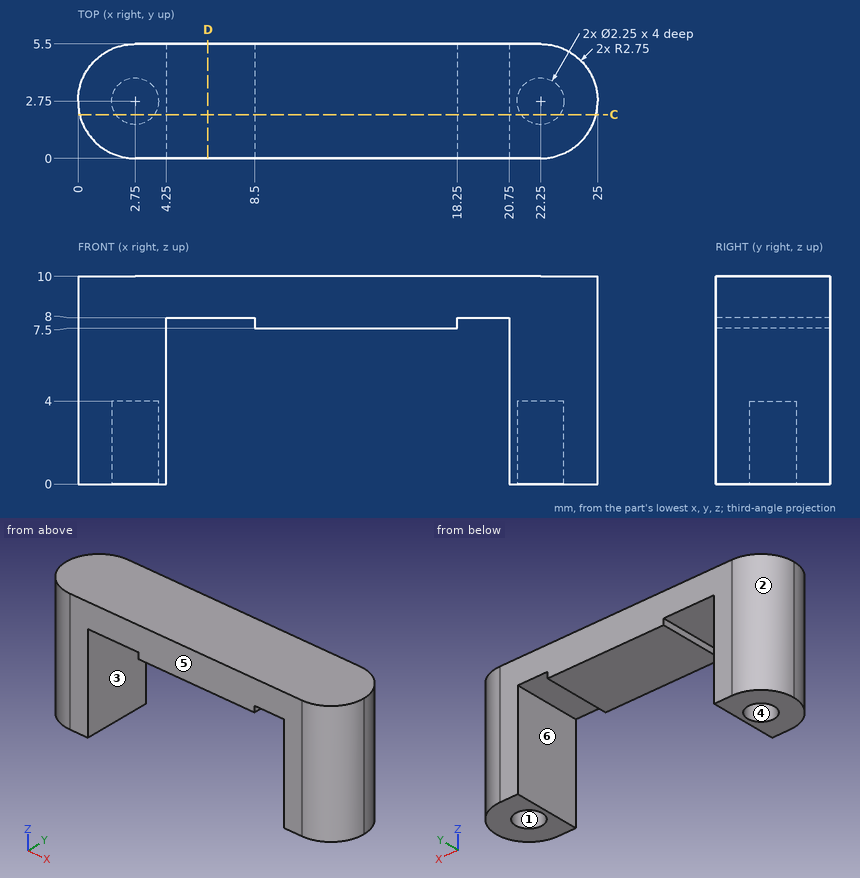
Can you work these out from the drawing? Everything is in mm from the part's minimum corner. A direction names the side the tool comes from. Give positions to 0.01 mm unless a question says otherwise; leave off trailing zeros. Loops run counter-clockwise (first coordinate to the right, second up) from the corner with the lowest first, then second, coordinate; pieces in that order, holes last. Notation, with made-up numbers: (-10.5, 73) -> (47.5, 73) arc R15 cw to (47.5, 82) -> close; hole circle Ø4 at (-26, -6). An arc over 180 degrees is marked (long way). Put each result on its own line as item: value.
(1) I'm going to push flat-ended pins straight in: pin 1 Ø1.3 at (x, y) = (7, 2.5) entering from -Z; pin 2 Ø1.8 at (x, y) = (2.75, 2.75) entering from -Z; pin 3 Ø1 at (y, z) = (2, 9) entering from -X. Where does each tip first touch, or does it pass through?
Computed:
pin 1: z = 8
pin 2: z = 4
pin 3: x = 0.01
(2) Please list where these lines run through material, in increasing order: probe 1 along X at (y, z) = (2.75, 1.85) (3 decimals); probe 2 along Y at (x, z) = (2.75, 1.05) (3 decimals); probe 3 along X at (y, z) = (2.15, 2.25). Write a range as [from, to].
Computed:
probe 1: [0, 1.625], [3.875, 4.25], [20.75, 21.125], [23.375, 25]
probe 2: [0, 1.625], [3.875, 5.5]
probe 3: [0.07, 1.8], [3.7, 4.25], [20.75, 21.3], [23.2, 24.93]
(3) Thinking about a two-plate mould opening in Y: for the marked faces 1, 2 and 3, which applies, pulls with the +Y half, pulls with the -Y half, needs draft (parallel to the pull), parting line crosses it, or undercut?
Computed:
face 1: undercut
face 2: pulls with the +Y half
face 3: needs draft
(4) Imagine slicing it at C-C on y = 2.1. Write out the boundary of the cut face in (x, z).
Computed:
outline: (0.08, 0) -> (1.83, 0) -> (1.83, 4) -> (3.67, 4) -> (3.67, 0) -> (4.25, 0) -> (4.25, 8) -> (8.5, 8) -> (8.5, 7.5) -> (18.25, 7.5) -> (18.25, 8) -> (20.75, 8) -> (20.75, 0) -> (21.33, 0) -> (21.33, 4) -> (23.17, 4) -> (23.17, 0) -> (24.92, 0) -> (24.92, 10) -> (0.08, 10) -> close
(5) For the marked faces 4, 5 and 6, which set-ups out of +Z, -Z, +X, -X, +Y, -Y let a thin tool reach every point of the face, with its end or its side?
Computed:
face 4: -Z
face 5: +Z, -Z, +X, -X, -Y
face 6: -Z, +Y, -Y
(6) Imagine slicing it at D-D on x = 6.25. Write out the boundary of the cut face in (y, z).
Computed:
outline: (0, 8) -> (5.5, 8) -> (5.5, 10) -> (0, 10) -> close
